from build123d import *

# Parameters (mm, degrees)
SKETCH1_W           = 42
SKETCH1_H           = 42
SKETCH1_R           = 1.5
BOSS_EXTRUDE1_DEPTH = 7
CUT_EXTRUDE1_DEPTH  = 5
SKETCH4_R           = 1.75
CUT_EXTRUDE3_DEPTH  = 2
SKETCH5_W           = 3
SKETCH5_H           = 10.8
CUT_EXTRUDE4_DEPTH  = 4
SKETCH6_R           = 3
CUT_EXTRUDE5_DEPTH  = 3
FILLET1_R           = 5
FILLET2_R           = 3


with BuildPart() as part:
    # Sketch1 → Boss-Extrude1 (new body)
    with BuildSketch(Plane(origin=(0, 0, 0), x_dir=(1, 0, 0), z_dir=(0, 1, 0))):
        Rectangle(SKETCH1_W, SKETCH1_H)
        with Locations(Location((-15.5, 15.5, 0), (0, 0, 270))):
            Circle(SKETCH1_R, mode=Mode.SUBTRACT)
        with Locations(Location((15.5, 15.5, 0), (0, 0, 270))):
            Circle(SKETCH1_R, mode=Mode.SUBTRACT)
        with Locations(Location((-15.5, -15.5, 0), (0, 0, 270))):
            Circle(SKETCH1_R, mode=Mode.SUBTRACT)
        with Locations(Location((15.5, -15.5, 0), (0, 0, 270))):
            Circle(SKETCH1_R, mode=Mode.SUBTRACT)
    extrude(amount=BOSS_EXTRUDE1_DEPTH)

    # Sketch2 → Cut-Extrude1 (cut)
    with BuildSketch(Plane(origin=(0, 7, 0), x_dir=(1, 0, 0), z_dir=(0, 1, 0))):
        Polygon((-11.5, 11.5), (-11.5, 21), (11.5, 21), (11.5, 11.5), (21, 11.5), (21, -11.5), (11.5, -11.5), (11.5, -21), (-11.5, -21), (-11.5, -11.5), (-21, -11.5), (-21, 11.5), align=None)
    extrude(amount=-CUT_EXTRUDE1_DEPTH, mode=Mode.SUBTRACT)

    # Sketch4 → Cut-Extrude3 (cut)
    with BuildSketch(Plane(origin=(0, 2, 0), x_dir=(1, 0, 0), z_dir=(0, 1, 0))):
        with Locations(Location((8, 8, 0), (0, 0, 270))):
            Circle(SKETCH4_R)
        with Locations(Location((8, -8, 0), (0, 0, 270))):
            Circle(SKETCH4_R)
        with Locations(Location((-8, -8, 0), (0, 0, 270))):
            Circle(SKETCH4_R)
        with Locations(Location((-8, 8, 0), (0, 0, 270))):
            Circle(SKETCH4_R)
    extrude(amount=-CUT_EXTRUDE3_DEPTH, mode=Mode.SUBTRACT)

    # Sketch5 → Cut-Extrude4 (cut)
    with BuildSketch(Plane(origin=(0, 2, 0), x_dir=(1, 0, 0), z_dir=(0, 1, 0))):
        with Locations((6.5, 0)):
            Rectangle(SKETCH5_W, SKETCH5_H)
        with Locations((-6.5, 0)):
            Rectangle(SKETCH5_W, SKETCH5_H)
    extrude(amount=-CUT_EXTRUDE4_DEPTH, mode=Mode.SUBTRACT)

    # Sketch6 → Cut-Extrude5 (cut)
    with BuildSketch(Plane.XZ):
        with Locations(Location((-15.5, 15.5, 0), (0, 0, 270))):
            Circle(SKETCH6_R)
        with Locations(Location((15.5, 15.5, 0), (0, 0, 270))):
            Circle(SKETCH6_R)
        with Locations(Location((15.5, -15.5, 0), (0, 0, 270))):
            Circle(SKETCH6_R)
        with Locations(Location((-15.5, -15.5, 0), (0, 0, 270))):
            Circle(SKETCH6_R)
    extrude(amount=-CUT_EXTRUDE5_DEPTH, mode=Mode.SUBTRACT)

    # Fillet1
    fillet1_edges = [part.edges().sort_by_distance(p)[0] for p in [
        (21, 3.5, 21),
        (-21, 3.5, 21),
        (-21, 3.5, -21),
        (21, 3.5, -21),
    ]]
    fillet(fillet1_edges, radius=FILLET1_R)

    # Fillet2
    fillet2_edges = [part.edges().sort_by_distance(p)[0] for p in [
        (11.5, 4.5, 11.5),
        (-11.5, 4.5, 11.5),
        (-11.5, 4.5, -11.5),
        (11.5, 4.5, -11.5),
    ]]
    fillet(fillet2_edges, radius=FILLET2_R)


solid = part.part
Verification items for the finished model (mm, model axes). A direction names the side the tool comes from. Round coordinates to 2 decimals unless told otherwise and drop trailing zeros. Write each loop counter-clockwise with the first axis right and the second up, starting at its lowest first coordinate (ties: lowest second). Pieces come first, ordered by that corner, then holes.
(1) Material ranges on line 1 (X direction, y = 1.65, z = -15.5); line 2 (X direction, y = 1, z = -3.5); line 3 (Z direction, x = 15.5, y = 5.95), recorded low to high.
Returned:
line 1: x = -21 to -18.5, -12.5 to 12.5, 18.5 to 21
line 2: x = -21 to -8, -5 to 5, 8 to 21
line 3: z = -21 to -17, -14 to -11.5, 11.5 to 14, 17 to 21
(2) Section check D-D (z = 12). Enter the section's corners in (x, y).
Returned:
outline: (-21, 0) - (21, 0) - (21, 7) - (12.84, 7) - (12.84, 2) - (-12.84, 2) - (-12.84, 7) - (-21, 7) - close
(3) Access from +Z, -Z, +X, -X, +Y, -Y to the whole of each face (thin tool, end or side, straight path). Record for faces 4 (the flat face through (-8, 1, 0)), 5 (the cylindrical face through (13.7, 1.5, 17.9)), 6 (the flat face through (18, 5, -11.5)).
Returned:
face 4: +Y, -Y
face 5: -Y
face 6: +X, -X, +Y
(4) Depth check by flat-ended pin: pin 1 Ø3 at (x, z) = (-15, 14.5) entering from -Y; pin 2 Ø2.5 at (x, z) = (-15.5, 15.5) entering from +Y; pin 3 Ø4 at (y, z) = (4, -19) entering from -X; pin 4 Ø4 at (x, z) = (8, -8) entering from +Y. Enter the tip coordinate at first touch or a pass-through.
Returned:
pin 1: stops at y = 3
pin 2: passes through
pin 3: stops at x = -20.9
pin 4: stops at y = 2
(5) Section check A-A (x = 5.5). Enter the section's corners in (y, z), plus the area to 3 significant figures.
Returned:
outline: (0, -21) - (2, -21) - (2, -5.4) - (0, -5.4) - close; (0, 5.4) - (2, 5.4) - (2, 21) - (0, 21) - close
area: 62.4 mm2
(6) Section check C-C (x = 15.5). Enter the section's corners in (y, z).
Returned:
outline: (0, -21) - (7, -21) - (7, -17) - (3, -17) - (3, -18.5) - (0, -18.5) - close; (0, -12.5) - (3, -12.5) - (3, -14) - (7, -14) - (7, -11.5) - (2, -11.5) - (2, 11.5) - (7, 11.5) - (7, 14) - (3, 14) - (3, 12.5) - (0, 12.5) - close; (0, 18.5) - (3, 18.5) - (3, 17) - (7, 17) - (7, 21) - (0, 21) - close
(7) Mould release check, pull along Z, two halves, no side actions. Record for faces 1 (the cylindrical face through (-15.43, 4.97, 14)), 2 (the flat face through (11.5, 5, -18)), 3 (the cylindrical face through (19, 4, -20)): pulls with the +Z half, pulls with the -Z half, needs draft (parallel to the pull), parting line crosses it, or undercut.
Returned:
face 1: undercut
face 2: needs draft
face 3: pulls with the -Z half
(8) Section check B-B (z = -15.5). Enter the section's corners in (x, y).
Returned:
outline: (-21, 0) - (-18.5, 0) - (-18.5, 3) - (-17, 3) - (-17, 7) - (-21, 7) - close; (-14, 3) - (-12.5, 3) - (-12.5, 0) - (12.5, 0) - (12.5, 3) - (14, 3) - (14, 7) - (11.5, 7) - (11.5, 2) - (-11.5, 2) - (-11.5, 7) - (-14, 7) - close; (17, 3) - (18.5, 3) - (18.5, 0) - (21, 0) - (21, 7) - (17, 7) - close
